Source: three-view drawing plus pictorial views. Frame: mm from the lowest corner of the part. A direction names the side the tool comes from. Give positions to 0.01 mm unless a question says otherwise; leave off trailing zeros. Order: outer loops, then holes, each group sorted by start corner. A loop starts at its lowest first (then second) coordinate and runs counter-clockwise, first axis right, second up. Notation, with made-up numbers: (48.25, 69) - (80.25, 69) arc R7 cw to (80.25, 75) - close; hole circle Ø10 at (26.25, 70). An arc over 180 degrees is marked (long way). Use CSV: the item, a comma, the result in double quotes.
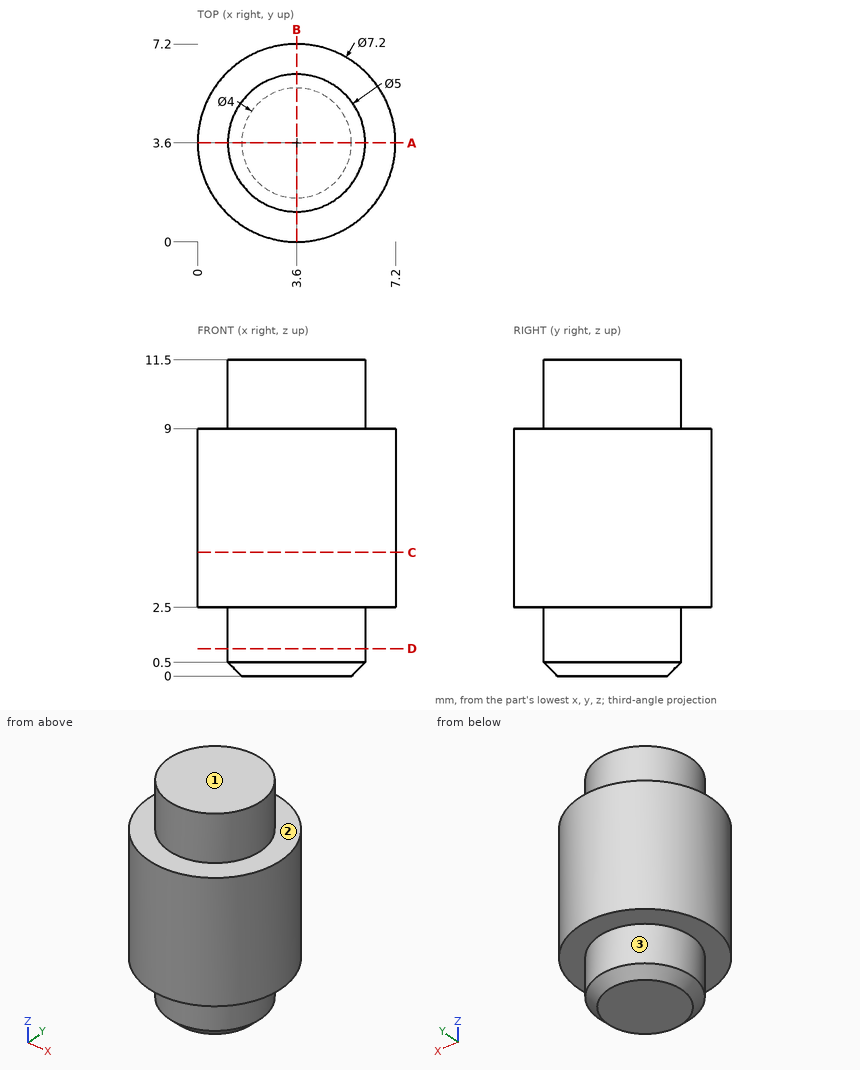
Item 1: Section A-A on y = 3.6. Return the cut outline in (x, z).
Filled in:
outline,"(0, 2.5) - (1.1, 2.5) - (1.1, 0.5) - (1.6, 0) - (5.6, 0) - (6.1, 0.5) - (6.1, 2.5) - (7.2, 2.5) - (7.2, 9) - (6.1, 9) - (6.1, 11.5) - (1.1, 11.5) - (1.1, 9) - (0, 9) - close"
Item 2: Section C-C on z = 4.5. Return the cut outline in (x, y).
Filled in:
outline,"circle Ø7.2 at (3.6, 3.6)"
Item 3: Material intervals for line 1 (Y direction, x = 3.75, z = 7.5); line 2 (Z direction, x = 6, y = 1); line 3 (Y direction, x = 5, z = 4.75), sorted ascending. Write a range as from..to.
Filled in:
line 1,"y = 0..7.2"
line 2,"z = 2.5..9"
line 3,"y = 0.28..6.92"
Item 4: Section D-D on z = 1. Return the cut outline in (x, y), then the cut area to 3 significant figures.
Filled in:
outline,"circle Ø5 at (3.6, 3.6)"
area,"19.6 mm2"
Item 5: First-contact query: pin 1 (2 mm diameter, centred on x = 2, z = 2, fed in from -Y); pin 2 (1 mm diameter, centred on y = 6.5, z = 2.5, fed in from -X). Flat tips, straight axial feed; report the tip coordinate or a pass-through.
Filled in:
pin 1,"stops at y = 0.08"
pin 2,"stops at x = 0.92"
Item 6: Set-up query: the marked faces 1, 2 and 3. Return all of +Z, -Z, +X, -X, +Y, -Y with unobstructed straight access to the full face (end or side cutting, diameter ignored); none if empty.
Filled in:
face 1,"+Z, +X, -X, +Y, -Y"
face 2,"+Z"
face 3,"-Z"
